```python
from build123d import *

# Parameters (mm, degrees)
BOSS_EXTRUDE1_DEPTH = 10
SKETCH2_R           = 6.25
CUT_EXTRUDE1_DEPTH  = 52.961524227


with BuildPart() as part:
    # Sketch1 → Boss-Extrude1 (new body)
    with BuildSketch(Plane.XY):
        with BuildLine():
            Line((0, 40), (0, 30))
            ThreePointArc((0, 30), (2.588190451, 30.340741737), (5, 31.339745962))
            Line((5, 31.339745962), (5, 40))
            Line((5, 40), (0, 40))
        make_face()
        with BuildLine():
            Line((0, 50), (0, 40))
            Line((0, 40), (5, 40))
            Line((5, 40), (5, 31.339745962))
            ThreePointArc((5, 31.339745962), (8.660254038, 35), (10, 40))
            ThreePointArc((10, 40), (7.071067812, 47.071067812), (0, 50))
        make_face()
        with BuildLine():
            ThreePointArc((-5, 31.339745962), (-2.588190451, 30.340741737), (0, 30))
            Line((0, 30), (0, 40))
            Line((0, 40), (-5, 40))
            Line((-5, 40), (-5, 31.339745962))
        make_face()
        with BuildLine():
            Line((-5, 40), (0, 40))
            Line((0, 40), (0, 50))
            ThreePointArc((0, 50), (-9.659258263, 42.588190451), (-5, 31.339745962))
            Line((-5, 31.339745962), (-5, 40))
        make_face()
        with BuildLine():
            Line((0, 30), (0, 10))
            ThreePointArc((0, 10), (2.588190451, 9.659258263), (5, 8.660254038))
            Line((5, 8.660254038), (5, 31.339745962))
            ThreePointArc((5, 31.339745962), (2.588190451, 30.340741737), (0, 30))
        make_face()
        with BuildLine():
            ThreePointArc((-5, 8.660254038), (-2.588190451, 9.659258263), (0, 10))
            Line((0, 10), (0, 30))
            ThreePointArc((0, 30), (-2.588190451, 30.340741737), (-5, 31.339745962))
            Line((-5, 31.339745962), (-5, 8.660254038))
        make_face()
        with BuildLine():
            Line((-5, 0), (0, 0))
            Line((0, 0), (0, 10))
            ThreePointArc((0, 10), (-2.588190451, 9.659258263), (-5, 8.660254038))
            Line((-5, 8.660254038), (-5, 0))
        make_face()
        with BuildLine():
            Line((0, 10), (0, 0))
            Line((0, 0), (5, 0))
            Line((5, 0), (5, 8.660254038))
            ThreePointArc((5, 8.660254038), (2.588190451, 9.659258263), (0, 10))
        make_face()
        with BuildLine():
            Line((5, 0), (0, 0))
            Line((0, 0), (-5, 0))
            Line((-5, 0), (-5, 8.660254038))
            ThreePointArc((-5, 8.660254038), (-5, -8.660254038), (10, 0))
            ThreePointArc((10, 0), (8.660254038, 5), (5, 8.660254038))
            Line((5, 8.660254038), (5, 0))
        make_face()
    extrude(amount=BOSS_EXTRUDE1_DEPTH)

    # Sketch2 → Cut-Extrude1 (cut, through all)
    with BuildSketch(Plane.XY.offset(10)):
        with Locations((0, 40)):
            Circle(SKETCH2_R)
        Circle(SKETCH2_R)
    extrude(amount=-CUT_EXTRUDE1_DEPTH, mode=Mode.SUBTRACT)


solid = part.part
```
The model under review builds one solid part; all positions refer to its coordinate system, in mm. A direction names the side the tool comes from. Coordinates: 2 decimals unless noted, no trailing zeros. Write each loop counter-clockwise with the first axis right and the second up, starting at its lowest first coordinate (ties: lowest second). Pieces come first, ordered by that corner, then holes. Notation, with made-up numbers: (33.25, -30.5) -> (50.25, -30.5) arc R21 ccw to (50.25, 2.5) -> close; hole circle Ø11 at (31.5, -38.75). An arc over 180 degrees is marked (long way). One line per item, written item: value. Start each with the question number.
Q1. To check wall thickness, follow probe 1 along Y at (x, z) = (0.25, 8.25) (3 decimals); probe 2 along Y at (x, z) = (-4.5, 6); probe 3 along X at (y, z) = (5.5, 5.75). State the ranges of each line that lie inside material, in increasing order.
Q2. Add section A-A, the plane z = 7.25. Give the boundary of the cut face in (x, y), then the cut area to 3 significant figures.
Q3. Add section C-C, the plane y = 15. Give the boundary of the cut face in (x, z), then the cut area to 3 significant figures.
Q4. The part is to be moulded in two halves that separate along Y. For faces 4 (the face through (0, 20, 0)), 5 (the face through (5.96, 1.88, 5.07)), say which applies: +Y half, -Y half, draft (parallel to the pull), parting line (faces both ways), or undercut.
Q5. Add section D-D, the plane x = 2. Give the boundary of the cut face in (y, z).
Q6. Clearance check with flat-ended pins moving along their axes: P1, Ø3, axis at x = 4, y = 40.5, coming from the -Z side; P2, Ø4, axis at x = 4, z = 3.5, coming from the +Y side; P3, Ø4, axis at y = 29.5, z = 9, coming from the -X side; P4, Ø3, axis at y = 20, z = 3, coming from the -X side. State where each tip first meets the part, or that it passes through.
Q7. Add section B-B, the plane x = -3.5. Give the boundary of the cut face in (y, z).
Q8. For faces 1 (the face through (-0.8, 46.2, 5.1)), 2 (the face through (-5, 20, 5)), 3 (the face through (5, 20, 5)), list the 3-axis set-ups (+Z, -Z, +X, -X, +Y, -Y) from which the entire face can be reached by the end or side of a thin tool; tool diameter is ignored.
Response:
1. probe 1: -9.997 to -6.245, 6.245 to 33.755, 46.245 to 49.997
1. probe 2: -8.93 to -4.34, 4.34 to 35.66, 44.34 to 48.93
1. probe 3: -8.35 to -2.97, 2.97 to 8.35
2. outline: (-5, 8.66) arc R10 ccw (long way) to (5, 8.66) -> (5, 31.34) arc R10 ccw (long way) to (-5, 31.34) -> close; hole circle Ø12.5 at (0, 0); hole circle Ø12.5 at (0, 40)
2. area: 592 mm²
3. outline: (-5, 0) -> (5, 0) -> (5, 10) -> (-5, 10) -> close
3. area: 100 mm²
4. face 4: draft
4. face 5: undercut
5. outline: (-9.8, 0) -> (-5.92, 0) -> (-5.92, 10) -> (-9.8, 10) -> close; (5.92, 0) -> (34.08, 0) -> (34.08, 10) -> (5.92, 10) -> close; (45.92, 0) -> (49.8, 0) -> (49.8, 10) -> (45.92, 10) -> close
6. P1: through
6. P2: y = 49.8
6. P3: x = -5.27
6. P4: x = -5
7. outline: (-9.37, 0) -> (-5.18, 0) -> (-5.18, 10) -> (-9.37, 10) -> close; (5.18, 0) -> (34.82, 0) -> (34.82, 10) -> (5.18, 10) -> close; (45.18, 0) -> (49.37, 0) -> (49.37, 10) -> (45.18, 10) -> close
8. face 1: +Z, -Z
8. face 2: +Z, -Z, -X
8. face 3: +Z, -Z, +X
